from build123d import *

# Parameters (mm, degrees)
SKETCH_1_W          = 49
SKETCH_1_H          = 90
SKETCH_1_R          = 1.75
EXTRUDE_1_DEPTH     = 3
FILLET_1_R          = 2
FILLET_2_R          = 5
CUT_EXTRUDE_1_DEPTH = 10


with BuildPart() as part:
    # 草图1 → 凸台-拉伸1 (new body)
    with BuildSketch(Plane(origin=(0, 0, 0), x_dir=(1, 0, 0), z_dir=(0, 1, 0))):
        Rectangle(SKETCH_1_W, SKETCH_1_H)
        Polygon((-4, 56), (-4, 45), (4, 45), (4, 56), (0, 56), align=None)
        with Locations((0, 49)):
            Circle(SKETCH_1_R, mode=Mode.SUBTRACT)
        Polygon((4, -45), (-4, -45), (-4, -56), (0, -56), (4, -56), align=None)
        with Locations((0, -49)):
            Circle(SKETCH_1_R, mode=Mode.SUBTRACT)
    extrude(amount=EXTRUDE_1_DEPTH)

    # 圆角1
    fillet_1_edges = [part.edges().sort_by_distance(p)[0] for p in [
        (-4, 1.5, -56),
        (4, 1.5, -56),
        (4, 1.5, 56),
        (-4, 1.5, 56),
    ]]
    fillet(fillet_1_edges, radius=FILLET_1_R)

    # 圆角2
    fillet_2_edges = [part.edges().sort_by_distance(p)[0] for p in [
        (-24.5, 1.5, 45),
        (-24.5, 1.5, -45),
        (24.5, 1.5, -45),
        (24.5, 1.5, 45),
    ]]
    fillet(fillet_2_edges, radius=FILLET_2_R)

    # 草图2 → 切除-拉伸1 (cut)
    with BuildSketch(Plane.XZ):
        with BuildLine():
            ThreePointArc((1.75, -28), (1.237436867, -26.762563133), (0, -26.25))
            Line((0, -26.25), (0, -28))
            Line((0, -28), (0, -29.75))
            ThreePointArc((0, -29.75), (1.237436867, -29.237436867), (1.75, -28))
        make_face()
        with BuildLine():
            Line((0, -28), (0, -26.25))
            ThreePointArc((0, -26.25), (-1.75, -28), (0, -29.75))
            Line((0, -29.75), (0, -28))
        make_face()
        with BuildLine():
            ThreePointArc((1.75, 28), (1.237436867, 29.237436867), (0, 29.75))
            Line((0, 29.75), (0, 28))
            Line((0, 28), (0, 26.25))
            ThreePointArc((0, 26.25), (1.237436867, 26.762563133), (1.75, 28))
        make_face()
        with BuildLine():
            Line((0, 28), (0, 29.75))
            ThreePointArc((0, 29.75), (-1.75, 28), (0, 26.25))
            Line((0, 26.25), (0, 28))
        make_face()
    extrude(amount=-CUT_EXTRUDE_1_DEPTH, mode=Mode.SUBTRACT)


solid = part.part
Work out the finished part from the listing and answer in its coordinate system (mm). A direction names the side the tool comes from. Give positions to 0.01 mm unless a question says otherwise; leave off trailing zeros. Loops run counter-clockwise (first coordinate to the right, second up) from the corner with the lowest first, then second, coordinate; pieces in that order, holes last. Notation, with made-up numbers: (18.25, 8) - (75.25, 8) arc R12 ccw to (75.25, 31) - close; hole circle Ø4 at (83, 23). An arc over 180 degrees is marked (long way). Answer in a Markdown table with one row per item. Add a question column.
Q1. The part is cut by section B-B (y = 1.45). Determine the outline of the cut face in (x, z).
Q2. The part is cut by section C-C (x = -6). Determine the outline of the cut face in (y, z).
Q3. A tool of negligible diameter and unlimited length cuts with its end or side. For faces 1 (the flat face through (4, 1, -49)), 2 (the flat face through (-12, 1, 45)), 3 (the flat face through (4, 1, 50)), 4 (the flat face through (-4, 1, -50)), from which of +Z, -Z, +X, -X, +Y, -Y can it reach the whole face along a straight path? Write none if from no direction.
Q4. The part is cut by section A-A (z = 49). Determine the outline of the cut face in (x, y).
Q5. Determine the mould class of faces 5 (the flat face through (12, 1, 45)), 6 (the cylindrical face through (3.4, 1.52, 55.43)), 7 (the flat face through (-4, 1, 49)), 8 (the cylindrical face through (-0.38, 1.48, -47.29)) for opening direction X: released by +X, released by -X, zero draft, split by the parting line, or undercut.
Q6. Each of these flat-tipped pins is pushed along its axis until it touches: P1, Ø0.9, axis at x = 8.5, y = 2, coming from the +Z side; P2, Ø1.5, axis at x = -10, y = 2, coming from the -Z side; P3, Ø2, axis at x = 0, z = -49, coming from the -Y side (3 decimals). Where does it stop, or does it pass through?
Q7. Consider line 1 along X through (y, z) = (1.7, 49); line 2 along Z through (x, y) = (1.5, 1.4); line 3 along X through (y, z) = (1.05, 27.5). Determine where each line is inside the solid, lowest interval first.
Solution:
| question | item | result |
|---|---|---|
| 1 | outline | (-24.5, -40) arc R5 ccw to (-19.5, -45) - (-4, -45) - (-4, -54) arc R2 ccw to (-2, -56) - (2, -56) arc R2 ccw to (4, -54) - (4, -45) - (19.5, -45) arc R5 ccw to (24.5, -40) - (24.5, 40) arc R5 ccw to (19.5, 45) - (4, 45) - (4, 54) arc R2 ccw to (2, 56) - (-2, 56) arc R2 ccw to (-4, 54) - (-4, 45) - (-19.5, 45) arc R5 ccw to (-24.5, 40) - close; hole circle Ø3.5 at (0, -49); hole circle Ø3.5 at (0, -28); hole circle Ø3.5 at (0, 28); hole circle Ø3.5 at (0, 49) |
| 2 | outline | (0, -45) - (3, -45) - (3, 45) - (0, 45) - close |
| 3 | face 1 | -Z, +X, +Y, -Y |
| 3 | face 2 | +Z, -X, +Y, -Y |
| 3 | face 3 | +Z, +X, +Y, -Y |
| 3 | face 4 | -Z, -X, +Y, -Y |
| 4 | outline | (-4, 0) - (-1.75, 0) - (-1.75, 3) - (-4, 3) - close; (1.75, 0) - (4, 0) - (4, 3) - (1.75, 3) - close |
| 5 | face 5 | zero draft |
| 5 | face 6 | released by +X |
| 5 | face 7 | released by -X |
| 5 | face 8 | undercut |
| 6 | P1 | stops at z = 45 |
| 6 | P2 | stops at z = -45 |
| 6 | P3 | passes through |
| 7 | line 1 | x = -4 to -1.75, 1.75 to 4 |
| 7 | line 2 | z = -56 to -49.9, -48.1 to -28.9, -27.1 to 27.1, 28.9 to 48.1, 49.9 to 56 |
| 7 | line 3 | x = -24.5 to -1.68, 1.68 to 24.5 |
